CAD build for the part. Positions are in the model's coordinates, mm. Face numbers are marked on the shaded views. A direction names the side the tool comes from. Round coordinates to 2 decimals unless told otherwise and drop trailing zeros. Loops run counter-clockwise (first coordinate to the right, second up) from the corner with the lowest first, then second, coordinate; pieces in that order, holes last. Notation, with made-up numbers: (87.5, 5) -> (112.5, 5) arc R33 ccw to (112.5, 42) -> close; hole circle Ø5 at (27.5, 10). An arc over 180 degrees is marked (long way). Answer as CSV lines item,"result".
```python
from build123d import *

# Parameters (mm, degrees)
F0_W          = 6.65
F0_H          = 12.3
F1_DEPTH      = 11
F2_R          = 1.525
F2_R_2        = 2
F3_DEPTH      = 2.5
F3_DEPTH_BACK = 3
F5_W          = 1.1
F5_H          = 1.35
F5_W_2        = 1.45
F5_H_2        = 1.3
F6_DEPTH      = 4.2


with BuildPart() as f1:
    # F0 (on Top) → F1 (new body)
    with BuildSketch(Plane.XY):
        with Locations((0, -0.62)):
            Rectangle(F0_W, F0_H)
    extrude(amount=F1_DEPTH)

    # F2 (on Top) → F3 (join, two sides)
    with BuildSketch(Plane.XY) as f3_sk:
        with Locations((0, 7)):
            Circle(F2_R)
        with Locations((0, -8.24)):
            Circle(F2_R_2)
    extrude(amount=-F3_DEPTH)
    extrude(f3_sk.sketch, amount=F3_DEPTH_BACK)

    # F5 (on face) → F6 (join, through all)
    with BuildSketch(Plane.XY.offset(11)):
        with Locations((0, 1.325)):
            Rectangle(F5_W, F5_H)
        with Locations((1.275, 0)):
            Rectangle(F5_W_2, F5_H_2)
        Rectangle(F5_W, F5_H_2)
        with Locations((-1.275, 0)):
            Rectangle(F5_W_2, F5_H_2)
        with Locations((0, -1.325)):
            Rectangle(F5_W, F5_H)
    extrude(amount=F6_DEPTH)


solid = f1.part
```
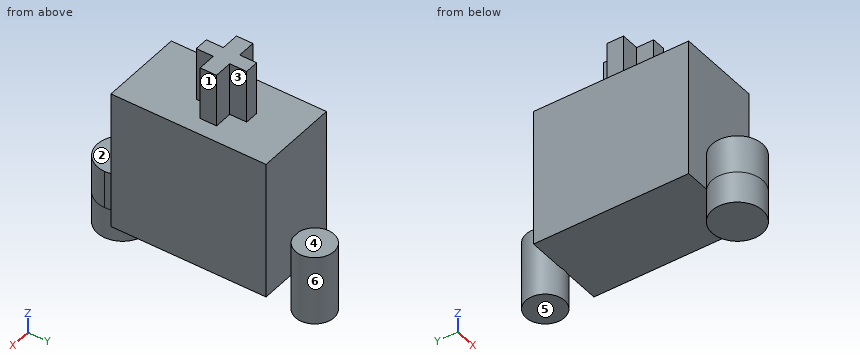
Q1. Probe L1, parallel to Y at x = 2, z = 4; L2, parallel to Z at x = -1.5, y = 0.25; L3, parallel to Z at x = 0.25, y = 4.25. List the from-to ranges inside material, lowest first. Write a range as [from, to].
Results:
L1,"[-6.77, 5.53]"
L2,"[0, 15.2]"
L3,"[0, 11]"
Q2. Two-plate mould, pull along Y, no slides. Class the marked faces 5 and 6: pulls with the +Y half, pulls with the -Y half, needs draft (parallel to the pull), parting line crosses it, or undercut.
Results:
face 5,"needs draft"
face 6,"undercut"
Q3. Slice it at A-A, the plane z = 11.5. Give the cut face in (x, y), and give its area (3 significant figures).
Results:
outline,"(-2, -0.65) -> (-0.55, -0.65) -> (-0.55, -2) -> (0.55, -2) -> (0.55, -0.65) -> (2, -0.65) -> (2, 0.65) -> (0.55, 0.65) -> (0.55, 2) -> (-0.55, 2) -> (-0.55, 0.65) -> (-2, 0.65) -> close"
area,"8.17 mm2"
Q4. Drop flat-ended pins along their axis: pin 1 Ø3 at (x, z) = (2, 0.5) entering from -Y; pin 2 Ø1.6 at (x, z) = (-1, 13.5) entering from +Y; pin 3 Ø1.2 at (x, z) = (1.5, 13.5) entering from +Y; pin 4 Ø1 at (y, z) = (5.5, 13) entering from +X. Give the stop position or say it passes through.
Results:
pin 1,"y = -10.18"
pin 2,"y = 2"
pin 3,"y = 0.65"
pin 4,"through"
Q5. Tool access for the marked faces 1, 2, 3 and 4: list every direction of +Z, -Z, +X, -X, +Y, -Y with a clear straight run to the whole face (end or side of a thin tool).
Results:
face 1,"+Z, +X, +Y, -Y"
face 2,"+Z, +X, -X, -Y"
face 3,"+Z, +X, +Y"
face 4,"+Z, +X, -X, +Y"
Q6. Slice it at B-B, the plane x = 0. Give the cut face in (y, z) (3 decimals).
Results:
outline,"(-10.24, -2.5) -> (-6.24, -2.5) -> (-6.24, 0) -> (5.475, 0) -> (5.475, -2.5) -> (8.525, -2.5) -> (8.525, 3) -> (5.53, 3) -> (5.53, 11) -> (2, 11) -> (2, 15.2) -> (-2, 15.2) -> (-2, 11) -> (-6.77, 11) -> (-6.77, 3) -> (-10.24, 3) -> close"
Q7. Slice it at C-C, the plane y = 2.25. Give the cut face in (x, z) (3 decimals).
Results:
outline,"(-3.325, 0) -> (3.325, 0) -> (3.325, 11) -> (-3.325, 11) -> close"
Q8. Slice it at D-D, the plane z = -0.25. Give the cut face in (x, y) (3 decimals), and give its area (3 significant figures).
Results:
outline,"circle Ø4 at (0, -8.24); circle Ø3.05 at (0, 7)"
area,"19.9 mm2"
